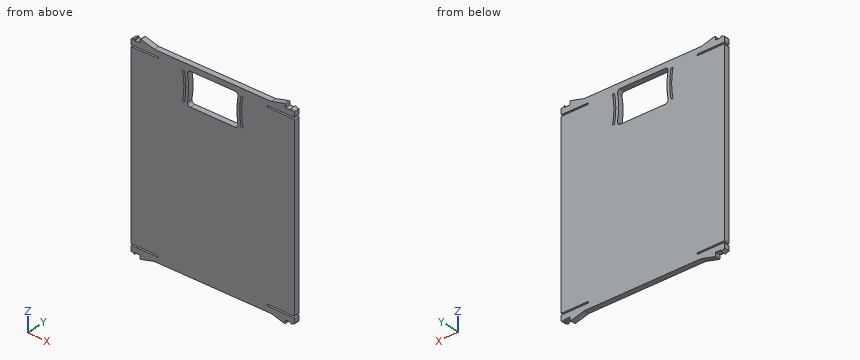
```python
from build123d import *

# Parameters (mm, degrees)
PAD008_DEPTH    = 2.8
FILLET001_R     = 0.4
POCKET004_DEPTH = 2.801


with BuildPart() as part:
    # Sketch008 (on Face4 of ShapeBinder007) → Pad008 (new body)
    with BuildSketch(Plane(origin=(0, 20.211282, 0), x_dir=(-1, 0, 0), z_dir=(0, 1, 0))):
        with BuildLine():
            Line((42.8, 63.127675), (42.8, 60.327675))
            Line((42.8, 60.327675), (28.8, 60.327675))
            ThreePointArc((28.8, 60.327675), (28.4, 59.927675), (28.8, 59.527675))
            Line((28.8, 59.527675), (42.8, 59.527675))
            Line((42.8, 59.527675), (42.8, -33.872325))
            Line((42.8, -33.872325), (28.8, -33.872325))
            ThreePointArc((28.8, -33.872325), (28.4, -34.272325), (28.8, -34.672325))
            Line((28.8, -34.672325), (42.8, -34.672325))
            Line((42.8, -34.672325), (42.8, -37.472325))
            Line((42.8, -37.472325), (40.8, -38.222325))
            Line((40.8, -38.222325), (40.8, -37.472325))
            Line((40.8, -37.472325), (38, -37.472325))
            Line((38, -39.472325), (38, -37.472325))
            Line((30.535898, -37.472325), (38, -39.472325))
            Line((-30.535898, -37.472325), (30.535898, -37.472325))
            Line((-38, -39.472325), (-30.535898, -37.472325))
            Line((-38, -37.472325), (-38, -39.472325))
            Line((-40.8, -37.472325), (-38, -37.472325))
            Line((-40.8, -38.222325), (-40.8, -37.472325))
            Line((-42.8, -37.472325), (-40.8, -38.222325))
            Line((-42.8, -37.472325), (-42.8, -34.672325))
            Line((-42.8, -34.672325), (-28.8, -34.672325))
            ThreePointArc((-28.8, -34.672325), (-28.4, -34.272325), (-28.8, -33.872325))
            Line((-28.8, -33.872325), (-42.8, -33.872325))
            Line((-42.8, -33.872325), (-42.8, 59.527675))
            Line((-28.8, 59.527675), (-42.8, 59.527675))
            ThreePointArc((-28.8, 59.527675), (-28.4, 59.927675), (-28.8, 60.327675))
            Line((-42.8, 60.327675), (-28.8, 60.327675))
            Line((-42.8, 60.327675), (-42.8, 63.127675))
            Line((-42.8, 63.127675), (-40.8, 63.877675))
            Line((-40.8, 63.877675), (-40.8, 63.127675))
            Line((-40.8, 63.127675), (-38, 63.127675))
            Line((-38, 65.127675), (-38, 63.127675))
            Line((-30.535898, 63.127675), (-38, 65.127675))
            Line((30.535898, 63.127675), (-30.535898, 63.127675))
            Line((38, 65.127675), (30.535898, 63.127675))
            Line((38, 63.127675), (38, 65.127675))
            Line((40.8, 63.127675), (38, 63.127675))
            Line((40.8, 63.877675), (40.8, 63.127675))
            Line((42.8, 63.127675), (40.8, 63.877675))
        make_face()
    extrude(amount=-PAD008_DEPTH)

    # Fillet001
    fillet001_edges = [part.edges().sort_by_distance(p)[0] for p in [
        (-38, 18.811282, -39.472325),
        (-42.8, 18.811282, -37.472325),
        (-42.8, 18.811282, -34.672325),
        (-42.8, 18.811282, -33.872325),
        (-42.8, 18.811282, 59.527675),
        (-42.8, 18.811282, 60.327675),
        (-42.8, 18.811282, 63.127675),
        (-38, 18.811282, 65.127675),
        (42.8, 18.811282, 59.527675),
        (42.8, 18.811282, 60.327675),
        (42.8, 18.811282, 63.127675),
        (38, 18.811282, 65.127675),
        (42.8, 18.811282, -33.872325),
        (42.8, 18.811282, -34.672325),
        (42.8, 18.811282, -37.472325),
        (38, 18.811282, -39.472325),
    ]]
    fillet(fillet001_edges, radius=FILLET001_R)

    # Sketch017 (on Face2 of Fillet001) → Pocket004 (cut, through all)
    with BuildSketch(Plane(origin=(0, 20.211282, 0), x_dir=(-1, 0, 0), z_dir=(0, 1, 0))):
        with BuildLine():
            ThreePointArc((-11.75, 60.327675), (-12.81066, 59.888335), (-13.25, 58.827675))
            ThreePointArc((-13.25, 58.827675), (-13.24452, 58.699573), (-13.22812, 58.572408))
            ThreePointArc((-13.22812, 45.082943), (-12.65, 51.827675), (-13.22812, 58.572408))
            ThreePointArc((-13.22812, 45.082943), (-13.24452, 44.955777), (-13.25, 44.827675))
            ThreePointArc((-13.25, 44.827675), (-12.81066, 43.767015), (-11.75, 43.327675))
            Line((11.75, 43.327675), (-11.75, 43.327675))
            ThreePointArc((11.75, 43.327675), (12.81066, 43.767015), (13.25, 44.827675))
            ThreePointArc((13.25, 44.827675), (13.24452, 44.955777), (13.22812, 45.082943))
            ThreePointArc((13.22812, 58.572408), (12.65, 51.827675), (13.22812, 45.082943))
            ThreePointArc((13.22812, 58.572408), (13.24452, 58.699573), (13.25, 58.827675))
            ThreePointArc((13.25, 58.827675), (12.81066, 59.888335), (11.75, 60.327675))
            Line((-11.75, 60.327675), (11.75, 60.327675))
        make_face()
        with BuildLine():
            ThreePointArc((-14.7587, 44.73481), (-14.09424, 51.827675), (-14.7587, 58.92054))
            ThreePointArc((-14.7587, 58.92054), (-15.342865, 59.318975), (-15.7413, 58.73481))
            ThreePointArc((-15.7413, 44.92054), (-15.09424, 51.827675), (-15.7413, 58.73481))
            ThreePointArc((-15.7413, 44.92054), (-15.342865, 44.336375), (-14.7587, 44.73481))
        make_face()
        with BuildLine():
            ThreePointArc((14.7587, 58.92054), (14.09424, 51.827675), (14.7587, 44.73481))
            ThreePointArc((14.7587, 44.73481), (15.342865, 44.336375), (15.7413, 44.92054))
            ThreePointArc((15.7413, 58.73481), (15.09424, 51.827675), (15.7413, 44.92054))
            ThreePointArc((15.7413, 58.73481), (15.342865, 59.318975), (14.7587, 58.92054))
        make_face()
    extrude(amount=-POCKET004_DEPTH, mode=Mode.SUBTRACT)


solid = part.part
```
Could you check a few things on this model? Use its own coordinates, in mm. Round coordinates to 2 decimals unless told otherwise and drop trailing zeros. Loops run counter-clockwise (first coordinate to the right, second up) from the corner with the lowest first, then second, coordinate; pieces in that order, holes last. Notation, with made-up numbers: (38, 30.5) - (57, 30.5) arc R10 cw to (57, 36.5) - close; hole circle Ø9 at (86.25, 16). An arc over 180 degrees is marked (long way). Answer in a Markdown table with one row per item. Add a question column.
(1) If we section it at B-B (y = 18.9): State how many separate pieces and enclosed holes the cut face has, plus the area to 3 significant figures.
(2) I need wall thicknesses on line 1 along Z through (x, y) = (39.5, 18.65); line 2 along X through (y, z) = (19.15, 53); line 3 along Z through (x, y) = (7, 18.65). Which ranges of each line are inside material? Lowest first, please.
(3) I'm going to push flat-ended pins straight in: pin 1 (1.4 mm diameter, centred on x = 39.5, y = 19, fed in from +Z); pin 2 (0.8 mm diameter, centred on x = 34.5, y = 19, fed in from +Z); pin 3 (0.8 mm diameter, centred on x = 3.5, y = 19, fed in from -Z). Where does each tip first touch, or does it pass through?
(4) If we section it at C-C (x = 21): Please give me the cut outline in (y, z), plus the area to 3 significant figures.
(5) If we section it at A-A (z = 53.5): Please give me the cut outline in (x, y), plus the area to 3 significant figures.
Model answer:
| question | item | result |
|---|---|---|
| 1 | separate pieces | 1 |
| 1 | enclosed holes | 3 |
| 1 | area | 8,130 mm² |
| 2 | line 1 | z = -37.47 to -34.67, -33.87 to 59.53, 60.33 to 63.13 |
| 2 | line 2 | x = -42.8 to -15.11, -14.11 to -12.67, 12.67 to 14.11, 15.11 to 42.8 |
| 2 | line 3 | z = -37.47 to 43.33, 60.33 to 63.13 |
| 3 | pin 1 | stops at z = 63.13 |
| 3 | pin 2 | stops at z = 64.3 |
| 3 | pin 3 | stops at z = -37.47 |
| 4 | outline | (17.41, -37.47) - (20.21, -37.47) - (20.21, 63.13) - (17.41, 63.13) - close |
| 4 | area | 282 mm² |
| 5 | outline | (-42.8, 17.41) - (-15.13, 17.41) - (-15.13, 20.21) - (-42.8, 20.21) - close; (-14.13, 17.41) - (-12.69, 17.41) - (-12.69, 20.21) - (-14.13, 20.21) - close; (12.69, 17.41) - (14.13, 17.41) - (14.13, 20.21) - (12.69, 20.21) - close; (15.13, 17.41) - (42.8, 17.41) - (42.8, 20.21) - (15.13, 20.21) - close |
| 5 | area | 163 mm² |
